Source: three-view drawing plus pictorial views. Frame: mm from the lowest corner of the part. Coordinates: 2 decimals unless noted, no trailing zeros. Loops run counter-clockwise (first coordinate to the right, second up) from the corner with the lowest first, then second, coordinate; pieces in that order, holes last. Notation, with made-up numbers: (9, 17.5) - (48, 17.5) arc R8 ccw to (48, 32.5) - close; hole circle Ø3 at (36, 28). An arc over 180 degrees is marked (long way). Return JSON: item names as keys, results as strings.
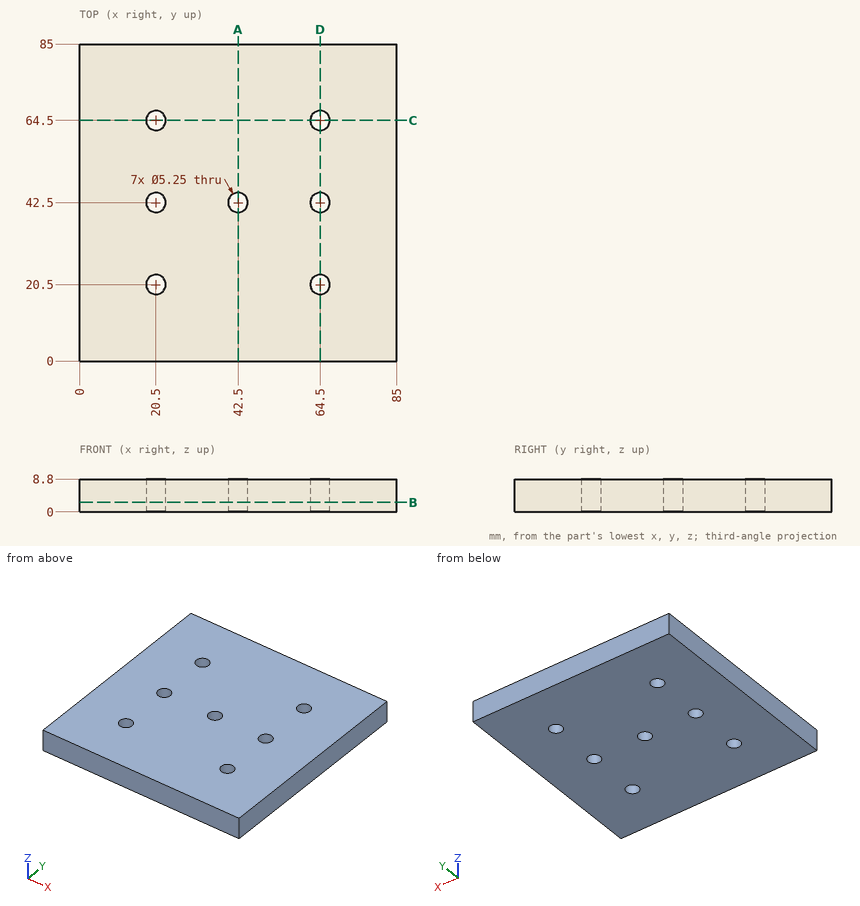
Item 1: Section query C-C, the plane y = 64.5. Return loops of the section in (x, z) (3 decimals).
Worked out:
{"outline": "(0, 0) - (17.875, 0) - (17.875, 8.8) - (0, 8.8) - close; (23.125, 0) - (61.875, 0) - (61.875, 8.8) - (23.125, 8.8) - close; (67.125, 0) - (85, 0) - (85, 8.8) - (67.125, 8.8) - close"}
Item 2: Section query B-B, the plane z = 2.5. Return loops of the section in (x, y) (3 decimals).
Worked out:
{"outline": "(0, 0) - (85, 0) - (85, 85) - (0, 85) - close; hole circle Ø5.25 at (20.5, 20.5); hole circle Ø5.25 at (20.5, 42.5); hole circle Ø5.25 at (20.5, 64.5); hole circle Ø5.25 at (42.5, 42.5); hole circle Ø5.25 at (64.5, 20.5); hole circle Ø5.25 at (64.5, 42.5); hole circle Ø5.25 at (64.5, 64.5)"}
Item 3: Ray query, probe 1 along X at (y, z) = (64.5, 4.25) (3 decimals); probe 2 along Y at (x, z) = (20.5, 2.5) (3 decimals); probe 3 along Y at (x, z) = (42.5, 4.25) (3 decimals). Return the intervals inside material, ascending. Write a range as from..to.
Worked out:
{"probe 1": "0..17.875, 23.125..61.875, 67.125..85", "probe 2": "0..17.875, 23.125..39.875, 45.125..61.875, 67.125..85", "probe 3": "0..39.875, 45.125..85"}
Item 4: Section query D-D, the plane x = 64.5. Return loops of the section in (y, z) (3 decimals), and give its area (3 significant figures).
Worked out:
{"outline": "(0, 0) - (17.875, 0) - (17.875, 8.8) - (0, 8.8) - close; (23.125, 0) - (39.875, 0) - (39.875, 8.8) - (23.125, 8.8) - close; (45.125, 0) - (61.875, 0) - (61.875, 8.8) - (45.125, 8.8) - close; (67.125, 0) - (85, 0) - (85, 8.8) - (67.125, 8.8) - close", "area": "609 mm^2"}
Item 5: Section query A-A, the plane x = 42.5. Return loops of the section in (y, z) (3 decimals).
Worked out:
{"outline": "(0, 0) - (39.875, 0) - (39.875, 8.8) - (0, 8.8) - close; (45.125, 0) - (85, 0) - (85, 8.8) - (45.125, 8.8) - close"}
